Here's how the part is built. I have some questions about the finished solid (model axes, mm). Face numbers are marked on the shaded views. A direction names the side the tool comes from. Round coordinates to 2 decimals unless told otherwise and drop trailing zeros. Loops run counter-clockwise (first coordinate to the right, second up) from the corner with the lowest first, then second, coordinate; pieces in that order, holes last. Notation, with made-up numbers: M 89.25,65.25 L 108.25,65.25 A33 ccw 108.25,94.25 Z; hole C 81,16 d4. An arc over 180 degrees is marked long. Answer as a JSON object with one key per item and string values.
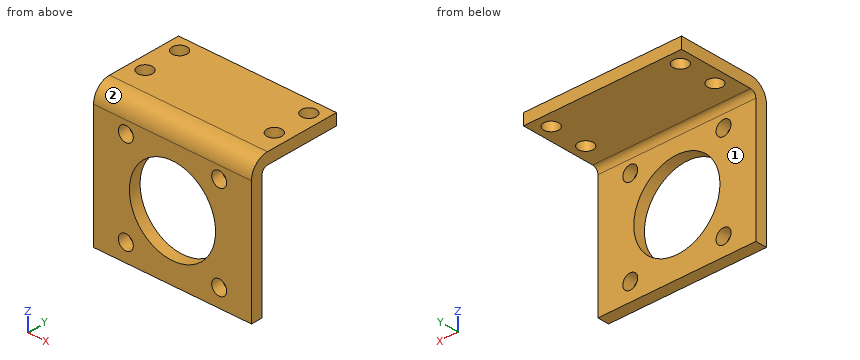
Autodesk Inventor part; units mm, degrees
ref_plane "YZ Plane" through (0, 0, 0) normal (1, 0, 0) x (0, 1, 0)
ref_plane "XZ Plane" through (0, 0, 0) normal (0, 1, 0) x (-1, 0, 0)
ref_plane "XY Plane" through (0, 0, 0) normal (0, 0, 1) x (1, 0, 0)
sketch "Skizze1" plane through (0, 0, 0) normal (1, 0, 0) x (0, 1, 0)
  line L0 (-153.8173, -10.7111) -> (-149.8173, -10.7111)
  line L1 (-149.8173, -10.7111) -> (-149.8173, 38.2889)
  line L2 (-149.8173, 38.2889) -> (-153.8173, 38.2889)
  line L3 (-153.8173, 38.2889) -> (-153.8173, -10.7111)
  line L4 (-153.8173, 38.2889) -> (-121.8173, 38.2889)
  line L5 (-121.8173, 38.2889) -> (-121.8173, 34.2889)
  line L6 (-121.8173, 34.2889) -> (-153.8173, 34.2889)
  line L7 (-153.8173, 34.2889) -> (-153.8173, 38.2889)
  point P0 (0, 0)
  point P1 (-149.8173, 34.2889)
  point P2 (-151.8173, -10.7111)
  dimension "d0" = 4
  dimension "d2" = 32
  dimension "d3" = 4
  dimension "d10" = 45
extrude "Extrusion1" add sketch "Skizze1" along normal blind 55
fillet "Rundung1" radius 2 1 edges at (27.5, -149.8173, 34.2889)
fillet "Rundung2" radius 6 1 edges at (27.5, -153.8173, 38.2889)
sketch "Skizze2" plane through (0, -149.8173, -10.7111) normal (0, 1, 0) x (1, 0, 0)
  line L0 (0, -45) -> (55, -45)
  line L1 (55, -43) -> (0, -43)
  line L2 (55, 0) -> (55, -43)
  point P0 (0, -10.7111)
  point P1 (43.75, -38.75)
  dimension "d9" = 4.25
  dimension "d24" = 11.25
hole "Bohrung1" at (43.75, -149.8173, 28.0389) direction (0, -1, 0) diameter 5.2 end through all
pattern_linear "Rechteckige Anordnung1" count 2 spacing 32.5 along (-1, 0, 0) count 2 spacing 32.5 along (0, 0, -1) of "Bohrung1"
sketch "Skizze3" plane through (55, -121.8173, 34.2889) normal (0, 0, -1) x (-1, 0, 0)
  line L0 (55, -28) -> (0, -28)
  line L1 (55, -26) -> (0, -26)
  line L2 (0, -26) -> (0, 0)
  point P0 (55, 121.8173)
  point P1 (5, -18)
  dimension "d27" = 5
  dimension "d28" = 10
hole "Bohrung2" at (50, -139.8173, 34.2889) direction (0, 0, 1) diameter 5.2 end through all
pattern_linear "Rechteckige Anordnung2" count 2 spacing 13 along (0, 1, 0) count 2 spacing 45 along (-1, 0, 0) of "Bohrung2"
sketch "Skizze4" plane through (0, -149.8173, -10.7111) normal (0, 1, 0) x (1, 0, 0)
  circle A0 centre (43.75, -38.75) radius 2.6 construction
  circle A1 centre (11.25, -6.25) radius 2.6 construction
  line L0 (43.75, -38.75) -> (11.25, -38.75) construction
  line L1 (11.25, -38.75) -> (11.25, -6.25) construction
  line L2 (11.25, -6.25) -> (43.75, -6.25) construction
  line L3 (43.75, -6.25) -> (43.75, -38.75) construction
  line L4 (43.75, -38.75) -> (11.25, -6.25) construction
  line L5 (43.75, -6.25) -> (11.25, -38.75) construction
  circle A2 centre (27.5, -22.5) radius 15
  point P0 (0, -10.7111)
  dimension "d42" = 30
extrude "Extrusion2" cut sketch "Skizze4" against normal through all
properties part number "TS_V1_Fallmagazin_Zylinderhalter_int"
Item 1: If I drill on L1, parallel to Z at x = 11.25, y = -151.8; L2, parallel to Z at x = 43.75, y = -152; L3, parallel to Y at x = 6, z = 35.5, over which ranges is the centre line in solid material (lowest first)? Write a range as from..to.
Solution:
{"L1": "z = -10.71..-7.06, -1.86..25.44, 30.64..36.78", "L2": "z = -10.71..-7.06, -1.86..25.44, 30.64..36.59", "L3": "y = -152.89..-142.22, -137.42..-129.22, -124.42..-121.82"}
Item 2: For P1, Ø4, axis at x = 50, y = -126.82, coming from the +Z side; P2, Ø1, axis at x = 20, z = 32, coming from the +Y side; P3, Ø7, axis at x = 5, y = -139.82, coming from the -Z side, each with a flat end and sliding along its axis, tell me the tip position at first contact or that it passes through.
Solution:
{"P1": "passes through", "P2": "stops at y = -149.81", "P3": "stops at z = 34.29"}
Item 3: I want a section at A-A on x = 11.25. List the corners of the cut face in (y, z) for me, plus the area to 3 significant figures.
Solution:
{"outline": "M -153.82,-10.71 L -149.82,-10.71 L -149.82,-7.06 L -153.82,-7.06 Z; M -153.82,-1.86 L -149.82,-1.86 L -149.82,25.44 L -153.82,25.44 Z; M -153.82,30.64 L -149.82,30.64 L -149.82,32.29 A2 cw -147.82,34.29 L -121.82,34.29 L -121.82,38.29 L -147.82,38.29 A6 ccw -153.82,32.29 Z", "area": "260 mm2"}
Item 4: For the marked faces 1 and 2, which set-ups out of +Z, -Z, +X, -X, +Y, -Y let a thin tool reach every point of the face, with its end or its side?
Solution:
{"face 1": "-Z, +X, -X, +Y", "face 2": "+Z, +X, -X, -Y"}
Item 5: I want a section at D-D on x = 27.5. List the corners of the cut face in (y, z) for me, plus the area to 3 significant figures.
Solution:
{"outline": "M -153.82,-10.71 L -149.82,-10.71 L -149.82,-3.21 L -153.82,-3.21 Z; M -153.82,26.79 L -149.82,26.79 L -149.82,32.29 A2 cw -147.82,34.29 L -121.82,34.29 L -121.82,38.29 L -147.82,38.29 A6 ccw -153.82,32.29 Z", "area": "181 mm2"}
Item 6: I want a section at C-C on z = -1. List the corners of the cut face in (x, y) for me, plus the area to 3 significant figures.
Solution:
{"outline": "M 0,-153.82 L 19.66,-153.82 L 19.66,-149.82 L 0,-149.82 Z; M 35.34,-153.82 L 55,-153.82 L 55,-149.82 L 35.34,-149.82 Z", "area": "157 mm2"}
Item 7: I want a section at B-B on y = -139. List the corners of the cut face in (x, z) for me, plus the area to 3 significant figures.
Solution:
{"outline": "M 0,34.29 L 2.53,34.29 L 2.53,38.29 L 0,38.29 Z; M 7.47,34.29 L 47.53,34.29 L 47.53,38.29 L 7.47,38.29 Z; M 52.47,34.29 L 55,34.29 L 55,38.29 L 52.47,38.29 Z", "area": "181 mm2"}
